Design review of the part built by this model. Coordinates are the model's own, in mm. Face numbers are marked on the shaded views. Round coordinates to 2 decimals unless told otherwise and drop trailing zeros. Loops run counter-clockwise (first coordinate to the right, second up) from the corner with the lowest first, then second, coordinate; pieces in that order, holes last. Notation, with made-up numbers: (18.5, -19.75) -> (45.5, -19.75) arc R20 ccw to (45.5, 10.25) -> close; hole circle Ø6 at (-30.75, 1). An arc over 180 degrees is marked (long way). Answer as CSV lines item,"result". Start each with the question number.
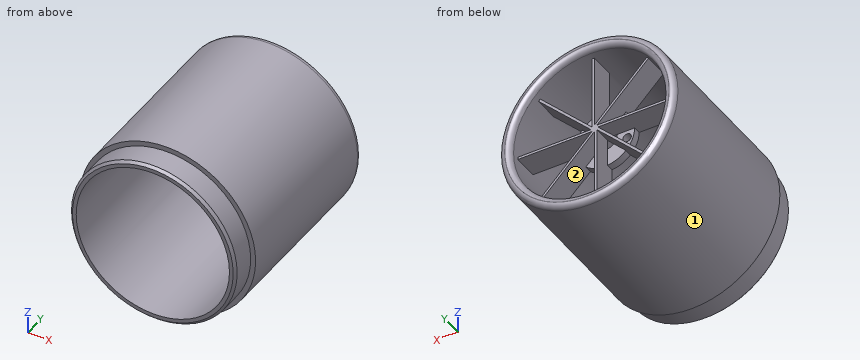
Autodesk Fusion 360 part; units mm, degrees
sketch "草图1" plane through (0, 0, 0) normal (0, 1, 0) x (1, 0, 0)
  circle A0 centre (0, 0) radius 35.5
  dimension "d1" = 71
extrude "拉伸1" add sketch "草图1" along normal blind 80
sketch "草图2" plane through (0, 80, 0) normal (0, 1, 0) x (-1, 0, 0)
  circle A0 centre (0, 0) radius 35.5
  circle A1 centre (0, 0) radius 31
  dimension "d4" = 62
extrude "拉伸2" cut sketch "草图2" against normal blind 90 contours A1
ref_plane "WorkPlane2" through (0, 75, 0) normal (0, 1, 0) x (-1, 0, 0)
sketch "Sketch5" plane through (0, 75, 0) normal (0, 1, 0) x (1, 0, 0)
  line L0 (0, 0) -> (31, 0)
  line L1 (31, 0) -> (31, 1)
  line L2 (31, 1) -> (0, 1)
  line L3 (0, 1) -> (0, 0)
  circle A0 centre (0, 0) radius 35.5
  circle A1 centre (0, 0) radius 35.5
  circle A2 centre (0, 0) radius 31
  dimension "d18" = 1
extrude "Extrude5" add sketch "Sketch5" against normal blind 10 contours L0 L2 L3 A2 picked at (10.328, 0.6667)
pattern_circular "C-Pattern1" count 8 over 360 about axis through (0, 1.75, 0) along (0, 1, 0) of "Extrude5"
sketch "Sketch6" plane through (0, 65, 0) normal (0, -1, 0) x (1, 0, 0)
  line L0 (1.4142, 0) -> (22.616, 21.2018)
  arc A0 (22.616, 21.2018) -> (21.9203, 21.9203) centre (0, 0) ccw
  line L1 (21.9203, 21.9203) -> (1, 1)
  line L2 (1, 1) -> (1, 30.9839)
  arc A1 (1, 30.9839) -> (0, 31) centre (0, 0) ccw
  line L3 (0, 31) -> (0, 1.4142)
  line L4 (0, 1.4142) -> (-21.2018, 22.616)
  arc A2 (-21.2018, 22.616) -> (-21.9203, 21.9203) centre (0, 0) ccw
  line L5 (-21.9203, 21.9203) -> (-1, 1)
  line L6 (-1, 1) -> (-30.9839, 1)
  arc A3 (-30.9839, 1) -> (-31, 0) centre (0, 0) ccw
  line L7 (-31, 0) -> (-1.4142, 0)
  line L8 (-1.4142, 0) -> (-22.616, -21.2018)
  arc A4 (-22.616, -21.2018) -> (-21.9203, -21.9203) centre (0, 0) ccw
  line L9 (-21.9203, -21.9203) -> (-1, -1)
  line L10 (-1, -1) -> (-1, -30.9839)
  arc A5 (-1, -30.9839) -> (0, -31) centre (0, 0) ccw
  line L11 (0, -31) -> (0, -1.4142)
  line L12 (0, -1.4142) -> (21.2018, -22.616)
  arc A6 (21.2018, -22.616) -> (21.9203, -21.9203) centre (0, 0) ccw
  line L13 (21.9203, -21.9203) -> (1, -1)
  line L14 (1, -1) -> (30.9839, -1)
  arc A7 (30.9839, -1) -> (31, 0) centre (0, 0) ccw
  line L15 (31, 0) -> (1.4142, 0)
  circle A8 centre (0, 0) radius 12
  dimension "d23" = 24
extrude "Extrude6" add sketch "Sketch6" against normal blind 3 contours L0 L1 L2 L3 L4 L5 L6 L7 L8 L9 L10 L11 L12 L13 L14 L15 A8 | L0 L15 A8 | L1 L2 A8 | L13 L14 A8 | L3 L4 A8 | L11 L12 A8 | L5 L6 A8 | L9 L10 A8 | L7 L8 A8
sketch "Sketch7" plane through (0, 65, 0) normal (0, -1, 0) x (1, 0, 0)
  line L0 (9.1629, 7.7487) -> (22.616, 21.2018)
  arc A0 (22.616, 21.2018) -> (21.9203, 21.9203) centre (0, 0) ccw
  line L1 (21.9203, 21.9203) -> (8.4853, 8.4853)
  arc A1 (8.4853, 8.4853) -> (1, 11.9583) centre (0, 0) ccw
  line L2 (1, 11.9583) -> (1, 30.9839)
  arc A2 (1, 30.9839) -> (0, 31) centre (0, 0) ccw
  line L3 (0, 31) -> (0, 12)
  arc A3 (0, 12) -> (-7.7487, 9.1629) centre (0, 0) ccw
  line L4 (-7.7487, 9.1629) -> (-21.2018, 22.616)
  arc A4 (-21.2018, 22.616) -> (-21.9203, 21.9203) centre (0, 0) ccw
  line L5 (-21.9203, 21.9203) -> (-8.4853, 8.4853)
  arc A5 (-8.4853, 8.4853) -> (-11.9583, 1) centre (0, 0) ccw
  line L6 (-11.9583, 1) -> (-30.9839, 1)
  arc A6 (-30.9839, 1) -> (-31, 0) centre (0, 0) ccw
  line L7 (-31, 0) -> (-12, 0)
  arc A7 (-12, 0) -> (-9.1629, -7.7487) centre (0, 0) ccw
  line L8 (-9.1629, -7.7487) -> (-22.616, -21.2018)
  arc A8 (-22.616, -21.2018) -> (-21.9203, -21.9203) centre (0, 0) ccw
  line L9 (-21.9203, -21.9203) -> (-8.4853, -8.4853)
  arc A9 (-8.4853, -8.4853) -> (-1, -11.9583) centre (0, 0) ccw
  line L10 (-1, -11.9583) -> (-1, -30.9839)
  arc A10 (-1, -30.9839) -> (0, -31) centre (0, 0) ccw
  arc A11 (0, -12) -> (7.7487, -9.1629) centre (0, 0) ccw
  line L11 (7.7487, -9.1629) -> (21.2018, -22.616)
  arc A12 (21.2018, -22.616) -> (21.9203, -21.9203) centre (0, 0) ccw
  line L12 (21.9203, -21.9203) -> (8.4853, -8.4853)
  arc A13 (8.4853, -8.4853) -> (11.9583, -1) centre (0, 0) ccw
  line L13 (11.9583, -1) -> (30.9839, -1)
  arc A14 (30.9839, -1) -> (31, 0) centre (0, 0) ccw
  arc A15 (12, 0) -> (9.1629, 7.7487) centre (0, 0) ccw
  circle A16 centre (0, 0) radius 5
  line L14 (0, -31) -> (0, -12)
  line L15 (31, 0) -> (12, 0)
  dimension "d26" = 10
extrude "Extrude7" cut sketch "Sketch7" against normal blind 3 contours A16
sketch "Sketch8" plane through (0, 65, 0) normal (0, -1, 0) x (1, 0, 0)
  circle A0 centre (0, 0) radius 5
  line L0 (9.1629, 7.7487) -> (22.616, 21.2018)
  arc A1 (22.616, 21.2018) -> (21.9203, 21.9203) centre (0, 0) ccw
  line L1 (21.9203, 21.9203) -> (8.4853, 8.4853)
  arc A2 (8.4853, 8.4853) -> (1, 11.9583) centre (0, 0) ccw
  line L2 (1, 11.9583) -> (1, 30.9839)
  arc A3 (1, 30.9839) -> (0, 31) centre (0, 0) ccw
  line L3 (0, 31) -> (0, 12)
  arc A4 (0, 12) -> (-7.7487, 9.1629) centre (0, 0) ccw
  line L4 (-7.7487, 9.1629) -> (-21.2018, 22.616)
  arc A5 (-21.2018, 22.616) -> (-21.9203, 21.9203) centre (0, 0) ccw
  line L5 (-21.9203, 21.9203) -> (-8.4853, 8.4853)
  arc A6 (-8.4853, 8.4853) -> (-11.9583, 1) centre (0, 0) ccw
  line L6 (-11.9583, 1) -> (-30.9839, 1)
  arc A7 (-30.9839, 1) -> (-31, 0) centre (0, 0) ccw
  line L7 (-31, 0) -> (-12, 0)
  arc A8 (-12, 0) -> (-9.1629, -7.7487) centre (0, 0) ccw
  line L8 (-9.1629, -7.7487) -> (-22.616, -21.2018)
  arc A9 (-22.616, -21.2018) -> (-21.9203, -21.9203) centre (0, 0) ccw
  line L9 (-21.9203, -21.9203) -> (-8.4853, -8.4853)
  arc A10 (-8.4853, -8.4853) -> (-1, -11.9583) centre (0, 0) ccw
  line L10 (-1, -11.9583) -> (-1, -30.9839)
  arc A11 (-1, -30.9839) -> (0, -31) centre (0, 0) ccw
  arc A12 (0, -12) -> (7.7487, -9.1629) centre (0, 0) ccw
  line L11 (7.7487, -9.1629) -> (21.2018, -22.616)
  arc A13 (21.2018, -22.616) -> (21.9203, -21.9203) centre (0, 0) ccw
  line L12 (21.9203, -21.9203) -> (8.4853, -8.4853)
  arc A14 (8.4853, -8.4853) -> (11.9583, -1) centre (0, 0) ccw
  line L13 (11.9583, -1) -> (30.9839, -1)
  arc A15 (30.9839, -1) -> (31, 0) centre (0, 0) ccw
  arc A16 (12, 0) -> (9.1629, 7.7487) centre (0, 0) ccw
  line L14 (-42.8424, -14.7518) -> (51.2572, 17.6493) construction
  line L15 (-13.299, 38.6232) -> (13.2323, -38.4293) construction
  circle A17 centre (0, 0) radius 9.5 construction
  circle A18 centre (0, 0) radius 8 construction
  line L16 (0, -31) -> (0, -12)
  line L17 (31, 0) -> (12, 0)
  dimension "d29" = 90
  dimension "d31" = 19
  dimension "d32" = 16
hole "Hole1" at (-2.6045, 65, 7.5641) at (8.9824, 65, 3.0929) at (2.6045, 65, -7.5641) at (-8.9824, 65, -3.0929) direction (0, 1, 0) diameter 3.4 depth 3 tip angle 118
fillet "Fillet2" radius 2.2 2 edges at (-33.0976, 80, 12.8373) (28.9021, 80, 11.2101)
sketch "Sketch9" plane through (0, 0, 0) normal (0, -1, 0) x (1, 0, 0)
  circle A0 centre (0, 0) radius 31
  circle A1 centre (0, 0) radius 35.5
  circle A2 centre (0, 0) radius 33.5
  dimension "d45" = 67
extrude "Extrude8" cut sketch "Sketch9" against normal blind 10 contours A1
chamfer "Chamfer1" distance 1 angle 45 1 edges at (-31.233, 0, -12.1141)
Q1. To check wall thickness, follow probe 1 along Z at (x, y) = (-1, 46.5); probe 2 along Z at (x, y) = (17, 67.5); probe 3 along Z at (x, y) = (28.5, 69.5). State the ranges of each line that lie inside material, in increasing order. Write a range as from..to.
Q2. Add section A-A, the plane y = 58. Give the boundary of the cut face in (x, z).
Q3. For pin 1 Ø8 at (x, z) = (8, -24) entering from +Y; pin 2 Ø5 at (x, y) = (18, 67.5) entering from +Z; pin 3 Ø2 at (x, y) = (25, 41.5) entering from +Z; pin 4 Ø6 at (x, z) = (10, -6.5) entering from +Y, all flat-tipped, find the tip position at first contact; note any pin that passes through.
Q4. Add section B-B, the plane x = 24. State how many separate pieces and enclosed holes the cut face has, and give its area (3 significant figures).
Q5. Mouldability with a two-part tool opening along X and no side actions: class the marked faces 1 and 2 as pulls with the +X half, pulls with the -X half, needs draft (parallel to the pull), parting line crosses it, or undercut.
Worked answers:
1,probe 1,"z = -35.49..-30.98, 30.98..35.49"
1,probe 2,"z = -31.16..-25.92, -18.41..-17, -1..0, 15.59..17, 25.92..31.16"
1,probe 3,"z = -21.17..-12.2, -1..0, 12.2..21.17"
2,outline,"circle Ø71 at (0, 0); hole circle Ø62 at (0, 0)"
3,pin 1,"passes through"
3,pin 2,"stops at z = 31.94"
3,pin 3,"stops at z = 26.16"
3,pin 4,"stops at y = 75"
4,separate pieces,"3"
4,enclosed holes,"0"
4,area,"993 mm^2"
5,face 1,"parting line crosses it"
5,face 2,"undercut"
